Design review of the part built by this model. Coordinates are the model's own, in mm. Face numbers are marked on the shaded views. A direction names the side the tool comes from. Give positions to 0.01 mm unless a question says otherwise; leave off trailing zeros. Order: outer loops, then holes, each group sorted by start corner. A loop starts at its lowest first (then second) coordinate and runs counter-clockwise, first axis right, second up.
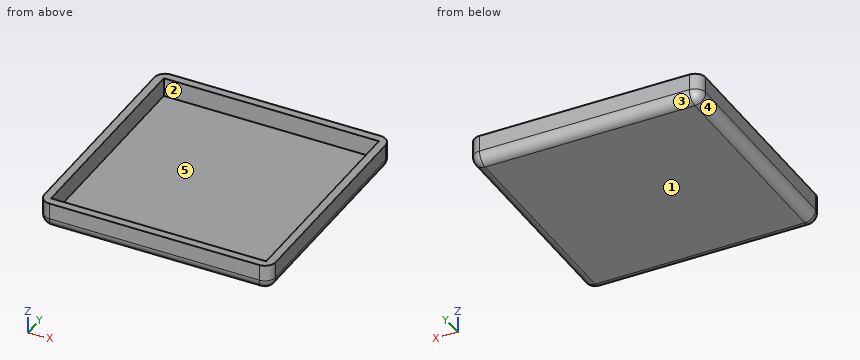
```python
from build123d import *

# Parameters (mm, degrees)
IZIM1_W                     = 43
IZIM1_H                     = 43
Y_KSEKLIK_EKSTR_ZYON1_DEPTH = 5
IZIM2_W                     = 40
IZIM2_H                     = 40
KES_EKSTR_ZYON1_DEPTH       = 3.5
RADYUS1_R                   = 2


with BuildPart() as part:
    # Çizim1 → Yükseklik-Ekstrüzyon1 (new body)
    with BuildSketch(Plane.XY.offset(5)):
        Rectangle(IZIM1_W, IZIM1_H)
    extrude(amount=-Y_KSEKLIK_EKSTR_ZYON1_DEPTH)

    # Çizim2 → Kes-Ekstrüzyon1 (cut)
    with BuildSketch(Plane.XY.offset(5)):
        Rectangle(IZIM2_W, IZIM2_H)
    extrude(amount=-KES_EKSTR_ZYON1_DEPTH, mode=Mode.SUBTRACT)

    # Radyus1
    radyus1_edges = [part.edges().sort_by_distance(p)[0] for p in [
        (21.5, 0, 0),
        (0, 21.5, 0),
        (-21.5, 0, 0),
        (-21.5, 21.5, 2.5),
        (21.5, 21.5, 2.5),
        (21.5, -21.5, 2.5),
        (-21.5, -21.5, 2.5),
        (0, -21.5, 0),
    ]]
    fillet(radyus1_edges, radius=RADYUS1_R)


solid = part.part
```
1. Machinability: for the marked faces 1 and 2, which of the approach directions +Z, -Z, +X, -X, +Y, -Y give a long, thin tool a straight path to every point of the face, cutting with its end or side? Answer none if there is none.
Recorded:
face 1: -Z, +X, -X, +Y, -Y
face 2: +Z
2. For line 1 along Y through (x, z) = (-2, 2.5); line 2 along Z through (x, y) = (2, -16.5), list the stretches that pass through material, from the lowest coordinate up.
Recorded:
line 1: y = -21.5 to -20, 20 to 21.5
line 2: z = 0 to 1.5
3. Take a section at A-A (z = 3.6). State the section outline as (x, y) points, then the cut area to 3 significant figures.
Recorded:
outline: (-21.5, -19.5) arc R2 ccw to (-19.5, -21.5) - (19.5, -21.5) arc R2 ccw to (21.5, -19.5) - (21.5, 19.5) arc R2 ccw to (19.5, 21.5) - (-19.5, 21.5) arc R2 ccw to (-21.5, 19.5) - close; hole (-20, -20) - (20, -20) - (20, 20) - (-20, 20) - close
area: 246 mm2
4. For pin 1 (3 mm diameter, centred on x = 4.5, y = 6, fed in from +Z), flat-tipped, find the tip position at first contact; note if it passes through.
Recorded:
pin 1: stops at z = 1.5
5. Draft analysis for pull direction Y (two halves, no side actions). For the marked faces 3, 4 and 5, state which applies: pulls with the +Y half, pulls with the -Y half, needs draft (parallel to the pull), parting line crosses it, or undercut.
Recorded:
face 3: pulls with the +Y half
face 4: needs draft
face 5: undercut
6. Take a section at B-B (y = 9.5). State the section outline as (x, z) points.
Recorded:
outline: (-21.5, 2) arc R2 ccw to (-19.5, 0) - (19.5, 0) arc R2 ccw to (21.5, 2) - (21.5, 5) - (20, 5) - (20, 1.5) - (-20, 1.5) - (-20, 5) - (-21.5, 5) - close
